Can you work these out from the model? Positions are in its coordinate system, mm. A direction names the side the tool comes from. Coordinates: 2 decimals unless noted, no trailing zeros. Order: outer loops, then holes, each group sorted by start corner. A loop starts at its lowest first (then second) coordinate and runs counter-clockwise, first axis right, second up. Notation, with made-up numbers: (59, -1.5) -> (98, -1.5) arc R18 ccw to (98, 10.5) -> close; hole circle Ø9 at (63, 24.5). An arc over 180 degrees is marked (long way). Write item = value, one per line.
```python
from build123d import *

# Parameters (mm, degrees)
F0_R     = 31.75
F1_DEPTH = 25.4


with BuildPart() as f1:
    # F0 (on Top) → F1 (new body)
    with BuildSketch(Plane.XY):
        Circle(F0_R)
        Polygon((-4.710587, -24.769592), (0, -16.610617), (4.710587, -24.769592), (0, -24.769592), align=None, mode=Mode.SUBTRACT)
        Polygon((-24.723618, 4.664613), (-16.644272, 0), (-16.564643, -0.045974), (-24.723618, -4.756561), (-24.723618, 0), align=None, mode=Mode.SUBTRACT)
        with BuildLine():
            ThreePointArc((-16.328571, -23.450125), (-20.205576, -20.205576), (-23.450125, -16.328571))
            ThreePointArc((-23.450125, -16.328571), (-23.86766, -9.760521), (-18.238986, -6.35))
            Line((-18.238986, -6.35), (-12.7, -6.35))
            ThreePointArc((-12.7, -6.35), (-8.209872, -8.209872), (-6.35, -12.7))
            Line((-6.35, -12.7), (-6.35, -18.238986))
            ThreePointArc((-6.35, -18.238986), (-9.760521, -23.86766), (-16.328571, -23.450125))
        make_face(mode=Mode.SUBTRACT)
        with BuildLine():
            ThreePointArc((6.35, -12.7), (8.209872, -8.209872), (12.7, -6.35))
            Line((12.7, -6.35), (18.238986, -6.35))
            ThreePointArc((18.238986, -6.35), (23.86766, -9.760521), (23.450125, -16.328571))
            ThreePointArc((23.450125, -16.328571), (20.205576, -20.205576), (16.328571, -23.450125))
            ThreePointArc((16.328571, -23.450125), (9.760521, -23.86766), (6.35, -18.238986))
            Line((6.35, -18.238986), (6.35, -12.7))
        make_face(mode=Mode.SUBTRACT)
        Polygon((16.564643, -0.045974), (16.644272, 0), (24.723618, 4.664613), (24.723618, 0), (24.723618, -4.756561), align=None, mode=Mode.SUBTRACT)
        with BuildLine():
            Line((-6.35, 18.238986), (-6.35, 12.7))
            ThreePointArc((-6.35, 12.7), (-8.209872, 8.209872), (-12.7, 6.35))
            Line((-12.7, 6.35), (-18.238986, 6.35))
            ThreePointArc((-18.238986, 6.35), (-23.86766, 9.760521), (-23.450125, 16.328571))
            ThreePointArc((-23.450125, 16.328571), (-20.205576, 20.205576), (-16.328571, 23.450125))
            ThreePointArc((-16.328571, 23.450125), (-9.760521, 23.86766), (-6.35, 18.238986))
        make_face(mode=Mode.SUBTRACT)
        with BuildLine():
            ThreePointArc((0, 6.35), (4.490128, 4.490128), (6.35, 0))
            ThreePointArc((6.35, 0), (4.490128, -4.490128), (0, -6.35))
            ThreePointArc((0, -6.35), (-4.490128, -4.490128), (-6.35, 0))
            ThreePointArc((-6.35, 0), (-4.490128, 4.490128), (0, 6.35))
        make_face(mode=Mode.SUBTRACT)
        with BuildLine():
            ThreePointArc((12.7, 6.35), (8.209872, 8.209872), (6.35, 12.7))
            Line((6.35, 12.7), (6.35, 18.238986))
            ThreePointArc((6.35, 18.238986), (9.760521, 23.86766), (16.328571, 23.450125))
            ThreePointArc((16.328571, 23.450125), (20.205576, 20.205576), (23.450125, 16.328571))
            ThreePointArc((23.450125, 16.328571), (23.86766, 9.760521), (18.238986, 6.35))
            Line((18.238986, 6.35), (12.7, 6.35))
        make_face(mode=Mode.SUBTRACT)
        Polygon((4.710587, 24.677645), (0, 16.518669), (-4.710587, 24.677645), (0, 24.677645), align=None, mode=Mode.SUBTRACT)
    extrude(amount=F1_DEPTH)


solid = f1.part
```
Item 1: If I drill on probe 1 along Y at (x, z) = (-7, 1.25); probe 2 along X at (y, z) = (14.5, 9.25); probe 3 along Y at (x, z) = (19.5, 12.25), over which ranges is the centre line in solid material (lowest first)?
A:
probe_1 = -30.97 to -21.04, -9.9 to 9.9, 21.04 to 30.97
probe_2 = -28.25 to -24.33, -6.35 to 6.35, 24.33 to 28.25
probe_3 = -25.06 to -20.89, -6.48 to -1.74, 1.65 to 6.48, 20.89 to 25.06
Item 2: If we mould it in two halves opening along Y, with no side actions, what happens to faces 3 (the cylindrical face through (-8.26, -8.16, 12.52)), 4 (the flat face through (-20.59, -2.37, 12.52)), 5 (the flat face through (7, 0, 0))? For each: pulls with the +Y half, pulls with the -Y half, needs draft (parallel to the pull), parting line crosses it, or undercut.
A:
face_3 = undercut
face_4 = undercut
face_5 = needs draft
Item 3: I want a section at A-A, the plane x = 15. Please give me the cut outline in (y, z), plus the area to 3 significant figures.
A:
outline = (-27.98, 0) -> (-24.16, 0) -> (-24.16, 25.4) -> (-27.98, 25.4) -> close; (-6.35, 0) -> (6.35, 0) -> (6.35, 25.4) -> (-6.35, 25.4) -> close; (24.16, 0) -> (27.98, 0) -> (27.98, 25.4) -> (24.16, 25.4) -> close
area = 517 mm2
Item 4: I'm going to push flat-ended pins straight in: P1, Ø3, axis at x = 19, z = 5.5, coming from the +Y side; P2, Ø5, axis at y = 14, z = 14, coming from the -X side; P3, Ø1.7, axis at x = 16, z = 15, coming from the -Y side. Where does each tip first touch, or does it pass through?
A:
P1 = 26.49
P2 = -29.59
P3 = -27.9
Item 5: I want a section at C-C, the plane x = -22. Please give me the cut outline in (y, z), plus the area to 3 significant figures.
A:
outline = (-22.89, 0) -> (-18.24, 0) -> (-18.24, 25.4) -> (-22.89, 25.4) -> close; (-7.58, 0) -> (-3.18, 0) -> (-3.18, 25.4) -> (-7.58, 25.4) -> close; (3.09, 0) -> (7.58, 0) -> (7.58, 25.4) -> (3.09, 25.4) -> close; (18.24, 0) -> (22.89, 0) -> (22.89, 25.4) -> (18.24, 25.4) -> close
area = 462 mm2
Item 6: I want a section at B-B, the plane y = 19. Please give me the cut outline in (x, z).
A:
outline = (-25.44, 0) -> (-21.34, 0) -> (-21.34, 25.4) -> (-25.44, 25.4) -> close; (-6.4, 0) -> (-1.43, 0) -> (-1.43, 25.4) -> (-6.4, 25.4) -> close; (1.43, 0) -> (6.4, 0) -> (6.4, 25.4) -> (1.43, 25.4) -> close; (21.34, 0) -> (25.44, 0) -> (25.44, 25.4) -> (21.34, 25.4) -> close
Item 7: I want a section at D-D, the plane y = 8.5. Please give me the cut outline in (x, z).
A:
outline = (-30.59, 0) -> (-23, 0) -> (-23, 25.4) -> (-30.59, 25.4) -> close; (-7.94, 0) -> (7.94, 0) -> (7.94, 25.4) -> (-7.94, 25.4) -> close; (23, 0) -> (30.59, 0) -> (30.59, 25.4) -> (23, 25.4) -> close
Item 8: For faces 1 (the flat face through (-2.39, -20.75, 12.52)), 2 (the flat face through (7, 0, 25.4)), which set-ups out of +Z, -Z, +X, -X, +Y, -Y let a thin tool reach every point of the face, with its end or its side?
A:
face_1 = +Z, -Z
face_2 = +Z, +X, -X, +Y, -Y
